CAD build for the part. Positions are in the model's coordinates, mm. A direction names the side the tool comes from. Coordinates: 2 decimals unless noted, no trailing zeros. Order: outer loops, then holes, each group sorted by start corner. A loop starts at its lowest first (then second) coordinate and runs counter-clockwise, first axis right, second up. Notation, with made-up numbers: M -37.5,-38 L -11.5,-38 A14 cw -11.5,-28 Z; hole C -15,-6 d9. An arc over 180 degrees is marked long. Write item = value, one per line.
Autodesk Inventor part; units mm, degrees
ref_plane "YZ Plane" through (0, 0, 0) normal (1, 0, 0) x (0, 1, 0)
ref_plane "XZ Plane" through (0, 0, 0) normal (0, 1, 0) x (-1, 0, 0)
ref_plane "XY Plane" through (0, 0, 0) normal (0, 0, 1) x (1, 0, 0)
sketch "Sketch1" plane through (0, 0, 0) normal (0, 0, 1) x (1, 0, 0)
  line L0 (-50, -100) -> (50, -100)
  line L1 (50, -100) -> (50, 100)
  line L2 (50, 100) -> (-50, 100)
  line L3 (-50, 100) -> (-50, -100)
  line L4 (-50, -100) -> (50, 100) construction
  line L5 (50, -100) -> (-50, 100) construction
  point P0 (0, 0)
  dimension "d0" = 100
  dimension "d1" = 200
extrude "Extrusion1" add sketch "Sketch1" along normal blind 5
sketch "Sketch2" plane through (-50, 100, 0) normal (0, 1, 0) x (1, 0, 0)
  line L0 (0, 0) -> (100, 0)
  line L1 (0, 0) -> (49.9986, 49.9986)
  line L2 (49.9986, 49.9986) -> (53.5341, 46.463)
  line L3 (53.5341, 46.463) -> (3.5355, -3.5355)
  line L4 (3.5355, -3.5355) -> (0, 0)
  line L5 (0, 0) -> (70.7086, 0) construction
  line L6 (100.108, -0.1109) -> (53.5341, 46.463)
  line L7 (53.5341, 46.463) -> (49.9986, 42.9275)
  line L8 (49.9986, 42.9275) -> (96.5724, -3.6464)
  line L9 (96.5724, -3.6464) -> (100.108, -0.1109)
  point P0 (50, 0)
  point P1 (49.9986, 42.9275)
  dimension "d4" = 45
  dimension "d5" = 5
  dimension "d6" = 5
extrude "Extrusion2" add sketch "Sketch2" against normal blind 30 contours L1 L2 L3 L0 | L0 L3 L4 | L8 L3 L6 L0 | L0 L6 L9 L8
sketch "Sketch6" plane through (0, 0, 5) normal (0, 0, 1) x (1, 0, 0)
  line L0 (4.9986, 75) -> (-5.0014, 75)
  line L1 (-25.0014, 55) -> (-25.0014, 45)
  line L2 (-5.0014, 25) -> (4.9986, 25)
  line L3 (24.9986, 45) -> (24.9986, 55)
  line L4 (24.9986, 75) -> (-25.0014, 25) construction
  line L5 (-25.0014, 75) -> (24.9986, 25) construction
  arc A0 (4.9986, 25) -> (24.9986, 45) centre (4.9986, 45) ccw
  arc A1 (24.9986, 55) -> (4.9986, 75) centre (4.9986, 55) ccw
  arc A2 (-5.0014, 75) -> (-25.0014, 55) centre (-5.0014, 55) ccw
  arc A3 (-25.0014, 45) -> (-5.0014, 25) centre (-5.0014, 45) ccw
  point P0 (0, 0)
  point P1 (-0.0014, 50)
  dimension "d21" = 50
  dimension "d22" = 50
  dimension "d23" = 20
extrude "Extrusion6" cut sketch "Sketch6" against normal blind 5
sketch "Sketch10" plane through (-50, 100, 5) normal (0, 1, 0) x (1, 0, 0)
  line L0 (0, 5) -> (7.0711, 5)
  line L1 (49.9986, 54.9986) -> (99.9971, 5)
  line L2 (0, 5) -> (49.9986, 54.9986)
  line L3 (49.9986, 54.9986) -> (46.463, 58.5341)
  line L4 (46.463, 58.5341) -> (-3.5355, 8.5355)
  line L5 (-3.5355, 8.5355) -> (0, 5)
  line L6 (100, 4.7812) -> (100, 0)
  line L7 (100, 4.7812) -> (49.9986, 54.9986)
  line L8 (49.9986, 54.9986) -> (53.5417, 58.5265)
  line L9 (53.5417, 58.5265) -> (103.5431, 8.3091)
  line L10 (103.5431, 8.3091) -> (100, 4.7812)
  line L11 (92.926, 5) -> (49.9986, 47.9275)
  line L12 (100, 0) -> (0, 0)
  line L13 (0, 0) -> (100, 0)
  point P0 (50, 5)
  dimension "d33" = 5
  dimension "d34" = 5
extrude "Extrusion9" add sketch "Sketch10" against normal blind 3
sketch "Sketch12" plane through (0, 0, 0) normal (0, 0, -1) x (-1, 0, 0)
  point P0 (0, 0)
sketch "Sketch13" plane through (0, 0, 0) normal (0, 0, -1) x (-1, 0, 0)
  line L0 (50, 100) -> (50, -100)
  line L1 (-50, -100) -> (-50, 97)
  line L2 (50, -100) -> (-50, -100)
  line L3 (-50, -100) -> (-50, 43.6313)
  line L4 (-50, 43.6313) -> (50, 43.6313)
  line L5 (50, 43.6313) -> (50, -100)
  point P0 (0, 0)
extrude "Extrusion10" cut sketch "Sketch13" against normal through all
properties part number "fixation_v08_ephys"
(1) Wall check: line 1 (Z direction, x = 21.5, y = 92); line 2 (Z direction, x = 32.5, y = 74.5); line 3 (X direction, y = 84.5, z = -14.5). Give the ranges that are in metal, low to high. Write a range as from..to.
Evaluation:
line_1 = -28.5..-21.43, 0..5
line_2 = -17.5..-10.43, 0..5
line_3 = -35.5..-28.43, 28.43..35.5
(2) Slice it at C-C, the plane z = -32. Write the cut outline in (x, y), then the cut area to 3 significant figures.
Evaluation:
outline = M -25.07,97 L -18,97 L -18,70 L -10.93,70 L -10.93,100 L -25.07,100 Z; M 10.93,70 L 18,70 L 18,97 L 24.98,97 L 24.98,100 L 10.93,100 Z
area = 466 mm²
(3) Pin check, flat tips, straight feed: pin 1 Ø4 at (y, z) = (68.5, 2) entering from +X; pin 2 Ø1.5 at (y, z) = (62, 3) entering from -X; pin 3 Ø25 at (x, z) = (14.5, -16) entering from -Y. Stop position of each tip, or through.
Evaluation:
pin_1 = 50
pin_2 = -50
pin_3 = 70
(4) Tool access for faces 4 (the face through (-18.987, 69.297, 2.535)), 5 (the face through (-25, 84, -25)), 6 (the face through (-21.165, 85.21, -21.764)): list every direction of +Z, -Z, +X, -X, +Y, -Y with a clear straight run to the whole face (end or side of a thin tool).
Evaluation:
face_4 = +Z, -Y
face_5 = -Z, -X, -Y
face_6 = +Y, -Y
(5) Slice it at D-D, the plane y = 62.5. Write the cut outline in (x, z), then the cut area to 3 significant figures.
Evaluation:
outline = M -50,0 L -23.54,0 L -23.54,5 L -50,5 Z; M 23.54,0 L 50,0 L 50,5 L 23.54,5 Z
area = 265 mm²
(6) Pull direction Z, two halves, no side cores. Call faces 1 (the face through (27, 97, -27)), 2 (the face through (1.75, 98.52, -51.74)), 3 (the face through (-1, 78, 0)): +Z half, -Z half, draft (parallel to the pull), parting line (faces both ways), or undercut.
Evaluation:
face_1 = draft
face_2 = -Z half
face_3 = undercut
(7) Slice it at B-B, the plane x = 39. Write the cut outline in (y, z), then the cut area to 3 significant figures.
Evaluation:
outline = M 43.63,0 L 100,0 L 100,5 L 43.63,5 Z; M 70,-11 L 97,-11 L 97,-17.92 L 100,-17.92 L 100,-3.93 L 70,-3.93 Z
area = 515 mm²
